Verification items for this drawing (mm, ordinates from the low corner). Coordinates: 2 decimals unless noted, no trailing zeros. Write each loop counter-clockwise with the first axis right and the second up, starting at its lowest first coordinate (ties: lowest second). Pieces come first, ordered by that corner, then holes. Notation, with made-up numbers: M 4,10.5 L 32,10.5 A20 cw 32,15.5 Z; hole C 64,65 d10. An arc over 180 degrees is marked long. Write each question's results on one line, items separated by ' | '.
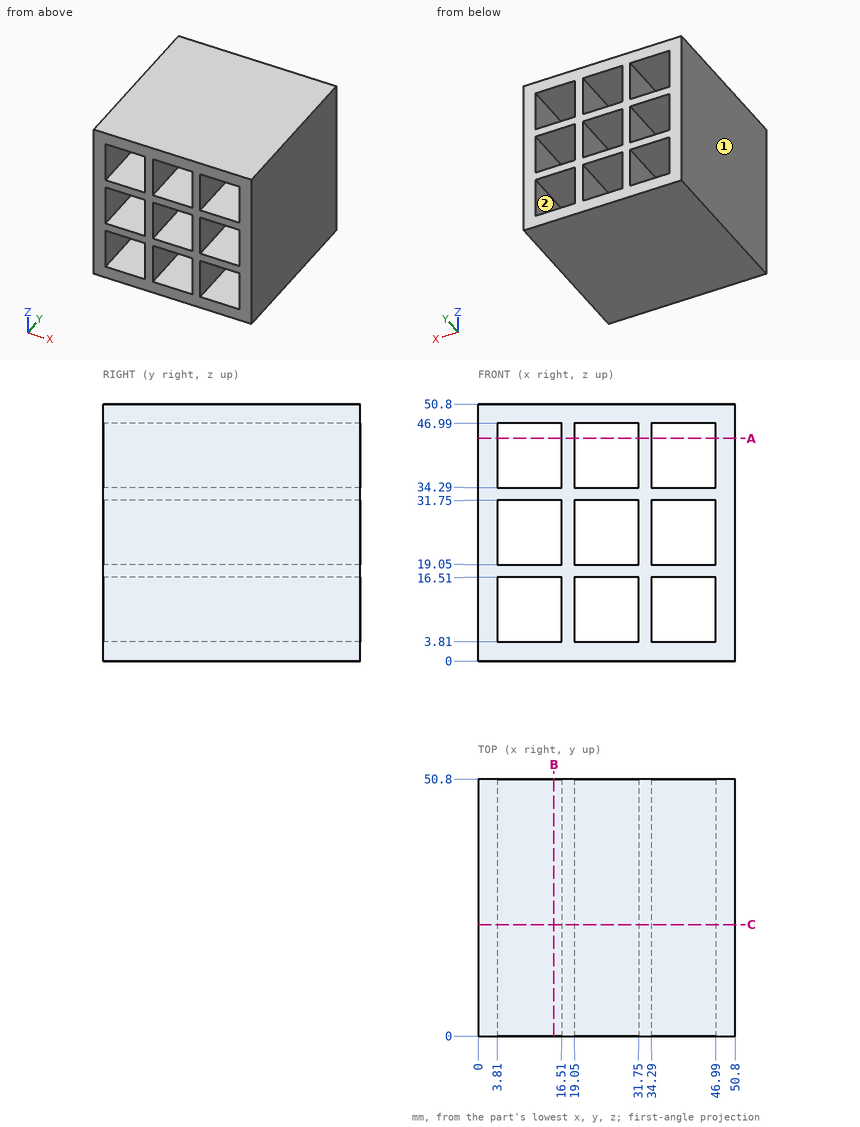
Q1. Mould release check, pull along X, two halves, no side actions. Record for the marked faces 1 and 2: pulls with the +X half, pulls with the -X half, needs draft (parallel to the pull), parting line crosses it, or undercut.
Geometry check:
face 1: pulls with the -X half | face 2: undercut
Q2. Sectioned sample at B-B on x = 15. Record the cut outline in (y, z), and give its area (3 significant figures).
Geometry check:
outline: M 0,0 L 50.8,0 L 50.8,3.81 L 0,3.81 Z; M 0,16.51 L 50.8,16.51 L 50.8,19.05 L 0,19.05 Z; M 0,31.75 L 50.8,31.75 L 50.8,34.29 L 0,34.29 Z; M 0,46.99 L 50.8,46.99 L 50.8,50.8 L 0,50.8 Z | area: 645 mm2
Q3. Scan line: probe 1 along Z at (x, y) = (11, 18). Record every from-to range of solid material in increasing order.
Geometry check:
probe 1: z = 0 to 3.81, 16.51 to 19.05, 31.75 to 34.29, 46.99 to 50.8
Q4. Sectioned sample at A-A on z = 44. Record the cut outline in (x, y), and give its area (3 significant figures).
Geometry check:
outline: M 0,0 L 3.81,0 L 3.81,50.8 L 0,50.8 Z; M 16.51,0 L 19.05,0 L 19.05,50.8 L 16.51,50.8 Z; M 31.75,0 L 34.29,0 L 34.29,50.8 L 31.75,50.8 Z; M 46.99,0 L 50.8,0 L 50.8,50.8 L 46.99,50.8 Z | area: 645 mm2
Q5. Sectioned sample at C-C on y = 22. Give the number of separate pieces and of enclosed holes in the cut face, and give its area (3 significant figures).
Geometry check:
separate pieces: 1 | enclosed holes: 9 | area: 1,130 mm2
